Verification items for this drawing (mm, ordinates from the low corner). Round coordinates to 2 decimals unless told otherwise and drop trailing zeros. Loops run counter-clockwise (first coordinate to the right, second up) from the corner with the lowest first, then second, coordinate; pieces in that order, holes last. Notation, with made-up numbers: (-27, 66) -> (23, 66) arc R26 ccw to (23, 97) -> close; hole circle Ø6 at (-5.75, 83.5). An arc over 180 degrees is marked (long way). Use a Markdown table: item, result. Add a question column.
Q1. Sectioned sample at B-B, the plane y = 20. Enter the section's corners in (x, z) (3 decimals), then the cut area to 3 significant figures.
Q2. Sectioned sample at A-A, the plane z = 24. Enter the section's corners in (x, y) (3 decimals).
Q3. Material ranges on L1, parallel to Z at x = 2, y = 7; L2, parallel to X at y = 34.5, z = 31; L3, parallel to Y at x = 2.5, z = 38, recorded low to high.
Q4. Sectioned sample at D-D, the plane y = 10.5. Enter the section's corners in (x, z), then the cut area to 3 significant figures.
Q5. Release check for a two-part mould opening along Z. For the marked faces 1, 2, 3 and 4 record: released by +Z, released by -Z, zero draft, split by the parting line, or undercut.
Q6. Sectioned sample at C-C, the plane x = 36. Enter the section's corners in (y, z) (3 decimals), then the cut area to 3 significant figures.
Q7. Gauge pin test, flat ends, axial feed: P1, Ø1, axis at x = 17.5, z = 17.5, coming from the -Y side; P2, Ø2, axis at x = 21, z = 25, coming from the +Y side; P3, Ø10, axis at x = 17.5, y = 28.5, coming from the +Z side. Record the tip position at first contact, or that the pin passes through.
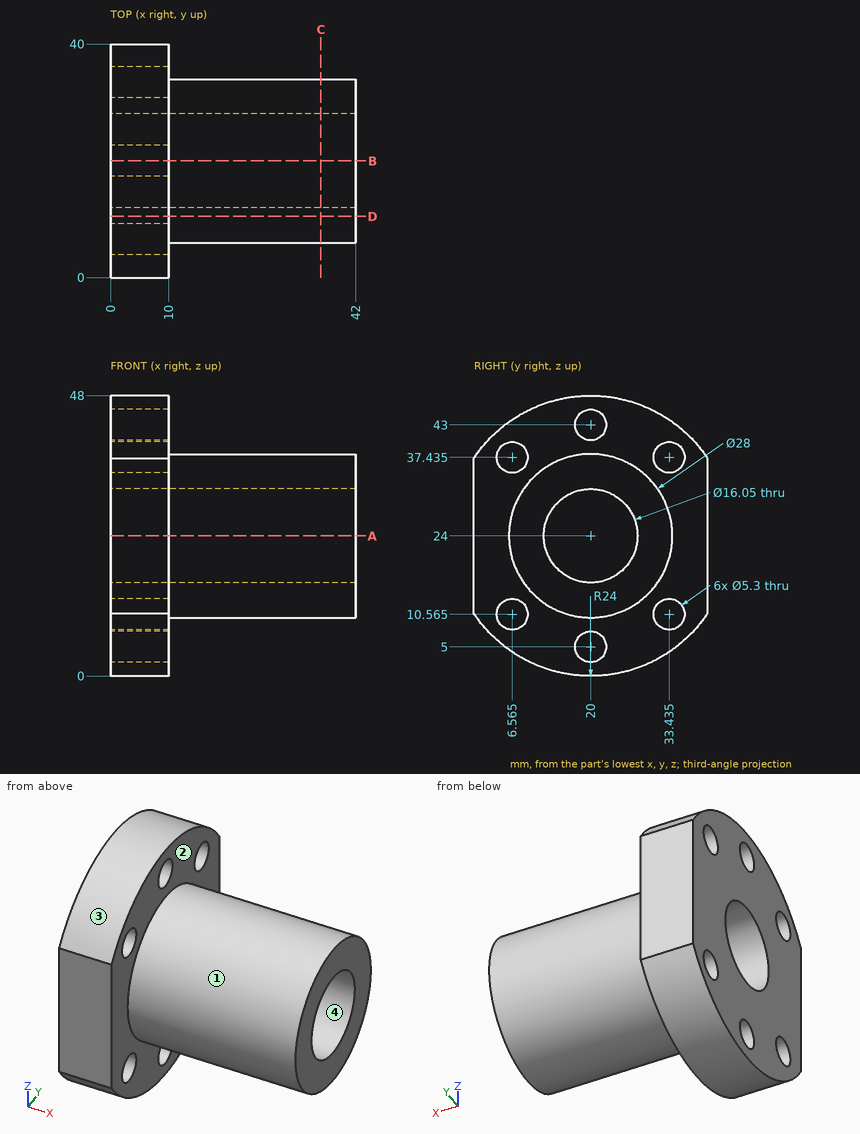
Values:
| question | item | result |
|---|---|---|
| 1 | outline | (0, 0) -> (10, 0) -> (10, 2.35) -> (0, 2.35) -> close; (0, 7.65) -> (10, 7.65) -> (10, 10) -> (42, 10) -> (42, 15.975) -> (0, 15.975) -> close; (0, 32.025) -> (42, 32.025) -> (42, 38) -> (10, 38) -> (10, 40.35) -> (0, 40.35) -> close; (0, 45.65) -> (10, 45.65) -> (10, 48) -> (0, 48) -> close |
| 1 | area | 596 mm^2 |
| 2 | outline | (0, 0) -> (10, 0) -> (10, 6) -> (42, 6) -> (42, 11.975) -> (0, 11.975) -> close; (0, 28.025) -> (42, 28.025) -> (42, 34) -> (10, 34) -> (10, 40) -> (0, 40) -> close |
| 3 | L1 | 3.83 to 7.95, 13.18 to 34.82, 40.05 to 44.17 |
| 3 | L2 | 0 to 10 |
| 3 | L3 | 0.51 to 3.98, 9.15 to 30.85, 36.02 to 39.49 |
| 4 | outline | (0, 1.96) -> (10, 1.96) -> (10, 13.72) -> (42, 13.72) -> (42, 34.28) -> (10, 34.28) -> (10, 46.04) -> (0, 46.04) -> close |
| 4 | area | 1,100 mm^2 |
| 5 | face 1 | split by the parting line |
| 5 | face 2 | zero draft |
| 5 | face 3 | released by +Z |
| 5 | face 4 | undercut |
| 6 | outline | circle Ø28 at (20, 24); hole circle Ø16.05 at (20, 24) |
| 6 | area | 413 mm^2 |
| 7 | P1 | y = 7.35 |
| 7 | P2 | y = 34 |
| 7 | P3 | z = 37.56 |
